Input: dimensioned drawing with shaded views. Units: mm. Origin: part minimum x, y, z. Coordinates: 2 decimals unless noted, no trailing zeros. Write each loop counter-clockwise with the first axis right and the second up, starting at its lowest first coordinate (ties: lowest second). Pieces come first, ordered by that corner, then holes. Notation, with made-up numbers: (-2, 64) -> (5, 64) arc R28 ccw to (5, 101) -> close; hole circle Ø9 at (20, 80). An arc over 180 degrees is marked (long way). One line per item, written item: value. Start each with the question number.
1. Section query D-D, the plane z = 10. Output: boundary loops of the cut face in (x, y) (1 decimal).
2. Section query B-B, the plane x = 20. State how many separate pieces and enclosed holes the cut face has, and give its area (3 significant figures).
3. Mould query, pull axis Z, two halves, no side actions, for the marked faces 1, 2, 3 and 4. Classes: released by +Z, released by -Z, zero draft, split by the parting line, or undercut.
4. First-contact query: P1, Ø1.9, axis at x = 20, z = 10.615, coming from the -Y side. Flat tip, straight axial feed; report the tip coordinate or a pass-through.
5. Line query: line 1 (Z direction, x = 10.5, y = 3.5) (1 decimal); line 2 (X direction, y = 3, z = 20); line 3 (X direction, y = 3, z = 10.5) (1 decimal). Output: solid intervals per line, ascending.
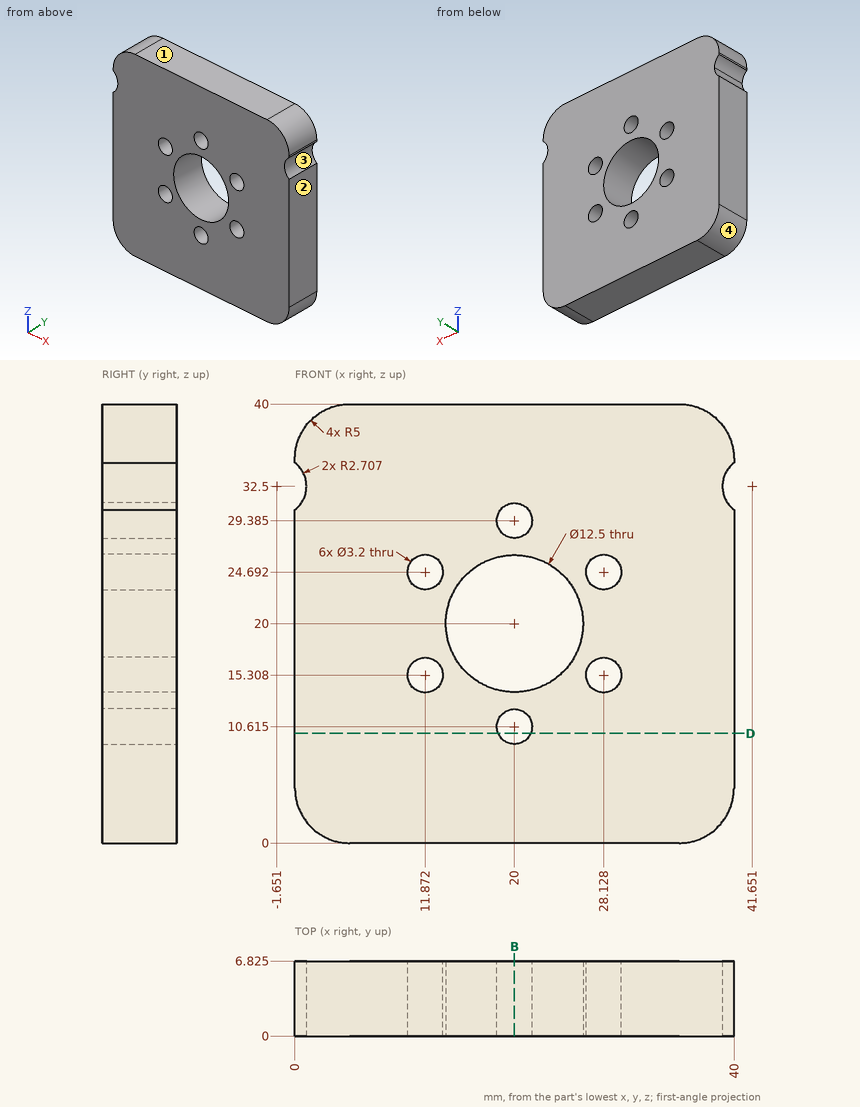
Computed values:
1. outline: (0, 0) -> (18.5, 0) -> (18.5, 6.8) -> (0, 6.8) -> close; (21.5, 0) -> (40, 0) -> (40, 6.8) -> (21.5, 6.8) -> close
2. separate pieces: 4
2. enclosed holes: 0
2. area: 144 mm²
3. face 1: released by +Z
3. face 2: zero draft
3. face 3: undercut
3. face 4: released by -Z
4. P1: passes through
5. line 1: z = 0 to 14.5, 16.1 to 23.9, 25.5 to 40
5. line 2: x = 0 to 13.75, 26.25 to 40
5. line 3: x = 0 to 18.4, 21.6 to 40
